```python
from build123d import *

# Parameters (mm, degrees)
BOSS_EXTRUDE2_DEPTH = 21
SKETCH2_W           = 12
SKETCH2_H           = 4.5
BOSS_EXTRUDE3_DEPTH = 15


with BuildPart() as part:
    # Sketch1 → Boss-Extrude2 (new body)
    with BuildSketch(Plane.XY):
        Polygon((4, 2), (4, 12), (33.684729064, 12), (33.684729064, 16), (-1, 16), (-1, 2), (-13, 2), (-13, -2), (13, -2), (13, 2), align=None)
    extrude(amount=BOSS_EXTRUDE2_DEPTH)

    # Sketch2 → Boss-Extrude3 (add)
    with BuildSketch(Plane.ZY.offset(13)):
        with Locations((10.5, 1.75)):
            Rectangle(SKETCH2_W, SKETCH2_H)
    extrude(amount=BOSS_EXTRUDE3_DEPTH)


solid = part.part
```
Check sheet for the modelled part. Datum: model origin and axes. Units: mm. A direction names the side the tool comes from. Round coordinates to 2 decimals unless told otherwise and drop trailing zeros. Write each loop counter-clockwise with the first axis right and the second up, starting at its lowest first coordinate (ties: lowest second). Pieces come first, ordered by that corner, then holes. Notation, with made-up numbers: M 56,-37.5 L 109,-37.5 A20 cw 109,-21.5 Z; hole C -9,40 d10. An arc over 180 degrees is marked long. Write item = value, one per line. Start each with the question number.
1. Section check C-C, the plane z = 7.5. Record the cut outline in (x, y), then the cut area to 3 significant figures.
2. Scan lines: line 1 (X direction, y = 3.5, z = 7.75); line 2 (X direction, y = 14.5, z = 12); line 3 (Y direction, x = 8, z = 9.25). Record each from-to range of solid material in increasing order. Write a range as [from, to].
3. Section check B-B, the plane x = -21. Record the cut outline in (y, z), then the cut area to 3 significant figures.
4. Tool access check on faces 5 (the flat face through (-20, 2, 4.5)), 6 (the flat face through (-20, 4, 10)), 7 (the flat face through (-7, 2, 10)), 8 (the flat face through (19, 12, 10)). Record the directions out of +Z, -Z, +X, -X, +Y, -Y that give a thin tool (end or side, any length) a straight path to the whole face; none if there is none.
5. Gauge pin test, flat ends, axial feed: pin 1 (3 mm diameter, centred on y = 5.5, z = 11, fed in from +X); pin 2 (9.5 mm diameter, centred on x = -21, z = 8, fed in from -Y); pin 3 (1.5 mm diameter, centred on x = 18.5, z = 18.5, fed in from -Y). Record the tip position at first contact, or that the pin passes through.
6. Release check for a two-part mould opening along Y. For faces 1 (the flat face through (17, 16, 10)), 2 (the flat face through (4, 7, 10)), 3 (the flat face through (9, 2, 10)), 4 (the flat face through (0, -2, 10)) record: pulls with the +Y half, pulls with the -Y half, needs draft (parallel to the pull), parting line crosses it, or undercut.
7. Section check A-A, the plane z = 17.5. Record the cut outline in (x, y), then the cut area to 3 significant figures.
8. Section check D-D, the plane y = 6.5. Record the cut outline in (x, z), then the cut area to 3 significant figures.
Results found:
q1.outline = M -28,-0.5 L -13,-0.5 L -13,-2 L 13,-2 L 13,2 L 4,2 L 4,12 L 33.68,12 L 33.68,16 L -1,16 L -1,2 L -13,2 L -13,4 L -28,4 Z
q1.area = 360 mm^2
q2.line_1 = [-28, -13], [-1, 4]
q2.line_2 = [-1, 33.68]
q2.line_3 = [-2, 2], [12, 16]
q3.outline = M -0.5,4.5 L 4,4.5 L 4,16.5 L -0.5,16.5 Z
q3.area = 54.0 mm^2
q4.face_5 = -Z, -X, +Y, -Y
q4.face_6 = +Z, -Z, -X, +Y
q4.face_7 = +Z, -Z, +Y
q4.face_8 = +Z, -Z, +X
q5.pin_1 = 4
q5.pin_2 = -0.5
q5.pin_3 = 12
q6.face_1 = pulls with the +Y half
q6.face_2 = undercut
q6.face_3 = undercut
q6.face_4 = pulls with the -Y half
q7.outline = M -13,-2 L 13,-2 L 13,2 L 4,2 L 4,12 L 33.68,12 L 33.68,16 L -1,16 L -1,2 L -13,2 Z
q7.area = 293 mm^2
q8.outline = M -1,0 L 4,0 L 4,21 L -1,21 Z
q8.area = 105 mm^2
